The listing builds one solid part. Answer for the finished solid, in the listing's coordinates (mm). Face numbers are marked on the shaded views. A direction names the side the tool comes from. Coordinates: 2 decimals unless noted, no trailing zeros. Order: outer loops, then holes, each group sorted by start corner. A loop starts at its lowest first (then second) coordinate and runs counter-clockwise, first axis right, second up. Notation, with made-up numbers: (-16, 3) -> (8, 3) arc R25 cw to (8, 16) -> close; hole circle Ø11 at (42, -39). An arc over 180 degrees is marked (long way). Answer in a Markdown table with one row per item.
```python
from build123d import *

# Parameters (mm, degrees)
F0_W     = 20
F0_H     = 20
F1_DEPTH = 4
F1_TAPER = 5
F2_R     = 2
F4_DEPTH = 1
F5_R     = 0.2
F7_DEPTH = 0.4
F8_R     = 0.1


with BuildPart() as f1:
    # F0 (on Top) → F1 (new body)
    with BuildSketch(Plane.XY):
        Rectangle(F0_W, F0_H)
    extrude(amount=F1_DEPTH, taper=F1_TAPER)

    # F2
    f2_edges = [f1.edges().sort_by_distance(p)[0] for p in [
        (9.650045, 0, 4),
        (0, 9.650045, 4),
        (-9.650045, 0, 4),
        (0, -9.650045, 4),
    ]]
    fillet(f2_edges, radius=F2_R)

    # F3 (on face) → F4 (join)
    with BuildSketch(Plane.XY.offset(4)):
        Polygon((3.8520088419, 3.9457110688), (0, 1.6323694726), (-3.8520088419, 3.9457110688), (-1.3217914384, 0), (-3.8520088419, -3.9457110688), (0, -1.6323694726), (3.8520088419, -3.9457110688), (1.3217914384, 0), align=None)
    extrude(amount=F4_DEPTH)

    # F5
    f5_edges = [f1.edges().sort_by_distance(p)[0] for p in [
        (2.5869, 1.972856, 5),
        (1.926004, 2.78904, 5),
        (-1.926004, 2.78904, 5),
        (-2.5869, 1.972856, 5),
        (-2.5869, -1.972856, 5),
        (-1.926004, -2.78904, 5),
        (1.926004, -2.78904, 5),
        (2.5869, -1.972856, 5),
        (-3.852009, 3.945711, 4.5),
        (-3.852009, -3.945711, 4.5),
        (3.852009, 3.945711, 4.5),
        (3.852009, -3.945711, 4.5),
    ]]
    fillet(f5_edges, radius=F5_R)

    # F6 (on face) → F7 (join)
    with BuildSketch(Plane.XY.offset(5)):
        Polygon((1.6986121191, 1.8877194962), (0, 0.5488963798), (-1.6986121191, 1.8877194962), (-0.4554191546, 0), (-1.6986121191, -1.8877194962), (0, -0.5488963798), (1.6986121191, -1.8877194962), (0.4554191546, 0), align=None)
    extrude(amount=F7_DEPTH)

    # F8
    f8_edges = [f1.edges().sort_by_distance(p)[0] for p in [
        (0.849306, 1.218308, 5.4),
        (-0.849306, 1.218308, 5.4),
        (-1.077016, 0.94386, 5.4),
        (-1.077016, -0.94386, 5.4),
        (-0.849306, -1.218308, 5.4),
        (0.849306, -1.218308, 5.4),
        (1.077016, -0.94386, 5.4),
        (1.077016, 0.94386, 5.4),
        (1.698612, 1.887719, 5.2),
        (1.698612, -1.887719, 5.2),
        (-1.698612, -1.887719, 5.2),
        (-1.698612, 1.887719, 5.2),
    ]]
    fillet(f8_edges, radius=F8_R)


solid = f1.part
```
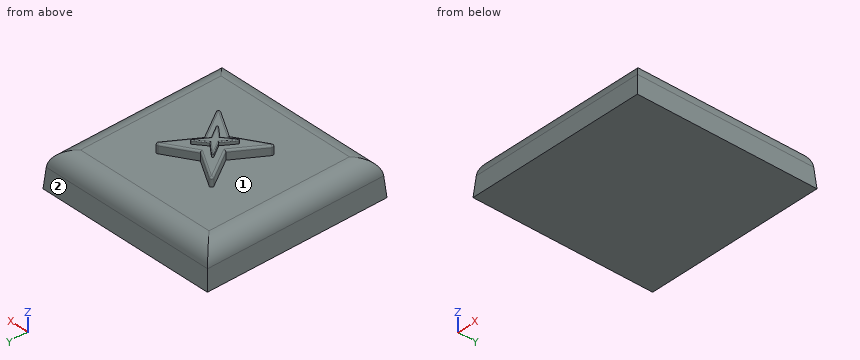
(1) A cutting plane is placed at D-D, the plane z = 2.6. Determine the outline of the cut face in (x, y), then the cut area to 3 significant figures.
Check values:
| item | result |
|---|---|
| outline | (-9.73, -9.73) -> (9.73, -9.73) -> (9.73, 9.73) -> (-9.73, 9.73) -> close |
| area | 378 mm² |
(2) A cutting plane is placed at A-A, the plane y = 5. Determine the outline of the cut face in (x, z).
Check values:
| item | result |
|---|---|
| outline | (-10, 0) -> (10, 0) -> (9.81, 2.17) arc R2 ccw to (7.82, 4) -> (-7.82, 4) arc R2 ccw to (-9.81, 2.17) -> close |
(3) A cutting plane is placed at B-B, the plane z = 4.4. Determine the outline of the cut face in (x, y).
Check values:
| item | result |
|---|---|
| outline | (-3.39, -3.23) arc R0.2 ccw to (-3.12, -3.51) -> (0, -1.63) -> (3.12, -3.51) arc R0.2 ccw to (3.39, -3.23) -> (1.32, 0) -> (3.39, 3.23) arc R0.2 ccw to (3.12, 3.51) -> (0, 1.63) -> (-3.12, 3.51) arc R0.2 ccw to (-3.39, 3.23) -> (-1.32, 0) -> close |
(4) Flat-ended cylindrical pins translate along their axes: pin 1 (1 mm diameter, centred on y = 6, z = 1.5, fed in from +X); pin 2 (5 mm diameter, centred on x = -4.5, y = -6, fed in from +Z); pin 3 (1 mm diameter, centred on y = 2.5, z = 4, fed in from -X). Find the tip coordinate at first contact, or state that the pin passes through.
Check values:
| item | result |
|---|---|
| pin 1 | x = 9.91 |
| pin 2 | z = 4 |
| pin 3 | x = -9.14 |
(5) Which of the six approach directions +Z, -Z, +X, -X, +Y, -Y give full straight-line access (tool end or side, diameter ignored) to the marked faces 1 and 2?
Check values:
| item | result |
|---|---|
| face 1 | +Z |
| face 2 | +Z, +X, -X, +Y |
(6) Find the intervals of material crossed by line 1 along Z through (x, y) = (-7.25, 9.25); line 2 along Z through (x, y) = (-7.5, 2.5); line 3 along Y through (x, z) = (2.75, 4.45), in increasing order. Write a range as from..to.
Check values:
| item | result |
|---|---|
| line 1 | 0..3.4 |
| line 2 | 0..4 |
| line 3 | -3.28..-2.23, 2.23..3.28 |
